Autodesk Inventor part; units mm, degrees
ref_plane "YZ Plane" through (0, 0, 0) normal (1, 0, 0) x (0, 1, 0)
ref_plane "XZ Plane" through (0, 0, 0) normal (0, 1, 0) x (-1, 0, 0)
ref_plane "XY Plane" through (0, 0, 0) normal (0, 0, 1) x (1, 0, 0)
sketch "Sketch1" plane through (0, 0, 0) normal (0, 0, 1) x (1, 0, 0)
  line L0 (0, 0) -> (80, 0)
  line L1 (80, 0) -> (80, -20)
  line L2 (80, -20) -> (0, -20)
  line L3 (0, -20) -> (0, 0)
  dimension "d0" = 80
  dimension "d1" = 20
extrude "Extrusion1" add sketch "Sketch1" along normal blind 7
sketch "Sketch2" plane through (0, 0, 7) normal (0, 0, 1) x (1, 0, 0)
  line L0 (0, 0) -> (80, 0)
  line L1 (80, 0) -> (80, -5)
  line L2 (80, -5) -> (0, -5)
  line L3 (0, -5) -> (0, 0)
  dimension "d4" = 80
  dimension "d5" = 5
extrude "Extrusion2" add sketch "Sketch2" along normal blind 7
sketch "Sketch3" plane through (0, -5, 7) normal (0, -1, 0) x (1, 0, 0)
  line L0 (0, -7) -> (0, 7)
  line L1 (0, 7) -> (80, 7)
  line L2 (80, 7) -> (80, 2)
  line L3 (80, 2) -> (0, 2)
  line L4 (0, 2) -> (0, 7)
  dimension "d8" = 80
  dimension "d9" = 5
extrude "Extrusion3" add sketch "Sketch3" along normal blind 7
sketch "Sketch6" plane through (0, 0, 14) normal (0, 0, 1) x (1, 0, 0)
  line L0 (80, 0) -> (0, 0)
  line L1 (1, -12) -> (79, -12)
  line L2 (15, 0) -> (65, 0)
  line L3 (65, 0) -> (65, -12)
  line L4 (65, -12) -> (15, -12)
  line L5 (15, -12) -> (15, 0)
  line L6 (0, -1) -> (0, -11)
  point P0 (79, 0)
  point P1 (1, 0)
  dimension "d28" = 50
  dimension "d29" = 15
extrude "Extrusion6" cut sketch "Sketch6" against normal blind 7
sketch "Sketch7" plane through (0, 0, 0) normal (0, 0, -1) x (-1, 0, 0)
  line L0 (0, 0) -> (-80, 0)
  line L1 (-80, 0) -> (-80, -35)
  line L2 (-80, -35) -> (0, -35)
  line L3 (0, -35) -> (0, 0)
  dimension "d38" = 80
  dimension "d39" = 35
extrude "Extrusion7" add sketch "Sketch7" along normal blind 7
sketch "Sketch8" plane through (0, 0, -7) normal (0, 0, -1) x (-1, 0, 0)
  circle A0 centre (-20, -17.75) radius 2.5
  line L0 (0, 0) -> (-80, 0)
  line L1 (0, -35) -> (0, 0)
  dimension "d42" = 5
  dimension "d43" = 17.75
  dimension "d44" = 20
extrude "Extrusion8" add sketch "Sketch8" along normal blind 5
sketch "Sketch9" plane through (0, 0, -7) normal (0, 0, -1) x (-1, 0, 0)
  circle A0 centre (-60, -17.75) radius 2.5
  line L0 (0, 0) -> (-80, 0)
  line L1 (-80, 0) -> (-80, -35)
  dimension "d47" = 5
  dimension "d48" = 17.75
  dimension "d49" = 20
extrude "Extrusion9" add sketch "Sketch9" along normal blind 5
chamfer "Chamfer5" distance 1 angle 45 30 edges at (0, -35, -3.5) (0, -27.5, 0) (0, -20, 3.5) (0, -12.5, 7) (40, -20, 7) (40, -35, 0) (0, 0, 3.5) (22.5, -17.75, -12) (62.5, -17.75, -12) (0, -6, 14) (72.5, -12, 14) (7.5, -12, 14) (15, -6, 14) (7.5, 0, 14) (7.5, -12, 9) (0, -12, 11.5) (15, -12, 11.5) (65, 0, 10.5) (65, -6, 14) (65, -12, 11.5) (72.5, -12, 9) (80, -12, 11.5) (80, -6, 14) (72.5, 0, 14) (80, 0, 3.5) (80, -35, -3.5) (80, -27.5, 0) (80, -20, 3.5) (80, -12.5, 7) (15, 0, 10.5)
properties part number "euro_box_center"
Model file for the job. Use its own axes, mm. A direction names the side the tool comes from. Coordinates: 2 decimals unless noted, no trailing zeros. Loops run counter-clockwise (first coordinate to the right, second up) from the corner with the lowest first, then second, coordinate; pieces in that order, holes last. Notation, with made-up numbers: (-28.5, 31.5) - (28.5, 31.5) arc R13 cw to (28.5, 43.5) - close; hole circle Ø8 at (50, 41.25). An arc over 180 degrees is marked (long way). Answer as a JSON object with one key per item and string values. Group by question number.
(1) Probe line 1 along Z through (x, y) = (76, -8.5); line 2 along Z through (x, y) = (60.5, -12); line 3 along Y through (x, z) = (8.5, 10.5). List the from-to ranges inside material, lowest first.
(2) Cut at A-A (y = -9.5). Give the cut face in (x, z).
(3) Two-plate mould, pull along X, no slides. Class faces 4 (the face through (15, -6, 11)), 5 (the face through (41, -35, -4)), 6 (the face through (0, -14, 1)): released by +X, released by -X, zero draft, split by the parting line, or undercut.
(4) Tool access for faces 1 (the face through (41, -20, 3)), 2 (the face through (73, -8, 9)), 3 (the face through (22.498, -17.86, -8.972)): list every direction of +Z, -Z, +X, -X, +Y, -Y with a clear straight run to the whole face (end or side of a thin tool).
(5) Cut at D-D (y = -3). Give the cut face in (x, z), then the cut area to 3 significant figures.
(6) Flat gauge pins, fed straight in: pin 1 (10 mm diameter, centred on y = -21.5, z = 10.5, fed in from -X); pin 2 (8 mm diameter, centred on x = 61.5, y = -29, fed in from +Z); pin 3 (1.8 mm diameter, centred on x = 70, y = -7, fed in from -Z); pin 4 (1.5 mm diameter, centred on y = -25.5, z = 1, fed in from -X). Where does each tip first touch, or does it go through?
(7) Cut at B-B (z = 11). Give the cut face in (x, y), then the cut area to 3 significant figures.
(8) Cut at C-C (x = 20). Give the cut face in (y, z).
Geometry says:
{
 "1": {"line 1": "z = -7 to 7, 9 to 14", "line 2": "z = -7 to 7", "line 3": "y = -12 to 0"},
 "2": {"outline": "(0, -7) - (80, -7) - (80, 6) - (79, 7) - (1, 7) - (0, 6) - close; (0, 9) - (15, 9) - (15, 13) - (14, 14) - (1, 14) - (0, 13) - close; (65, 9) - (80, 9) - (80, 13) - (79, 14) - (66, 14) - (65, 13) - close"},
 "3": {"face 4": "undercut", "face 5": "zero draft", "face 6": "released by -X"},
 "4": {"face 1": "+Z, +X, -X, -Y", "face 2": "+X, -X, -Y", "face 3": "-Z"},
 "5": {"outline": "(0, -7) - (80, -7) - (80, 13) - (79, 14) - (66, 14) - (65, 13) - (65, 7) - (15, 7) - (15, 13) - (14, 14) - (1, 14) - (0, 13) - close", "area": "1,330 mm^2"},
 "6": {"pin 1": "stops at x = 0.17", "pin 2": "stops at z = 0", "pin 3": "stops at z = -7", "pin 4": "passes through"},
 "7": {"outline": "(0, -11) - (1, -12) - (14, -12) - (15, -11) - (15, -1) - (14, 0) - (1, 0) - (0, -1) - close; (65, -11) - (66, -12) - (79, -12) - (80, -11) - (80, -1) - (79, 0) - (66, 0) - (65, -1) - close", "area": "356 mm^2"},
 "8": {"outline": "(-35, -7) - (-20.25, -7) - (-20.25, -11) - (-19.25, -12) - (-16.25, -12) - (-15.25, -11) - (-15.25, -7) - (0, -7) - (0, 7) - (-19, 7) - (-20, 6) - (-20, 0) - (-34, 0) - (-35, -1) - close"}
}
